from build123d import *

# Parameters (mm, degrees)
SKETCH1_W                = 36.8554
SKETCH1_H                = 17.1196
SKETCH1_W_2              = 19.8882
SKETCH1_H_2              = 6.985
SKETCH1_W_3              = 11.8237
SKETCH1_H_3              = 7.62
BOSS_EXTRUDE1_DEPTH      = 11.684
BOSS_EXTRUDE1_2_DEPTH    = 11.684
SKETCH3_R                = 1.4605
CUT_EXTRUDE8_DEPTH       = 140.210429827
SKETCH4_R                = 1.4605
CUT_EXTRUDE9_DEPTH       = 18.034
CUT_EXTRUDE11_DEPTH      = 38.1
SKETCH6_R                = 1.4605
CUT_EXTRUDE12_DEPTH      = 16.3195
CUT_EXTRUDE13_DEPTH      = 140.210429862
CUT_EXTRUDE13_DEPTH_BACK = 140.210429862
SKETCH7_R                = 1.9685
CUT_EXTRUDE14_DEPTH      = 7.62


with BuildPart() as part:
    # Sketch1 → Boss-Extrude1 (new body)
    with BuildSketch(Plane(origin=(0, 0, 0), x_dir=(1, 0, 0), z_dir=(0, 1, 0))):
        with BuildLine():
            Line((-25.4, 37.231859639), (-67.6656, 37.231859639))
            Line((-67.6656, 37.231859639), (-86.5378, 37.231859639))
            Line((-86.5378, 37.231859639), (-130.704860186, 33.167859639))
            Line((-130.704860186, 33.167859639), (-133.6294, 28.523199453))
            Line((-133.6294, 28.523199453), (-133.6294, 5.586999453))
            Line((-133.6294, 5.586999453), (-128.984739814, 2.662459639))
            Line((-128.984739814, 2.662459639), (-96.664183529, -1.34664073))
            ThreePointArc((-96.664183529, -1.34664073), (-60.341965715, -8.501620237), (-25.4, -20.730940361))
            Line((-25.4, -20.730940361), (-25.4, 37.231859639))
        make_face()
        with Locations((-111.1123, 17.953259639)):
            Rectangle(SKETCH1_W, SKETCH1_H, mode=Mode.SUBTRACT)
        with Locations((-76.367777447, 27.363959639)):
            Rectangle(SKETCH1_W_2, SKETCH1_H_2, mode=Mode.SUBTRACT)
        with Locations((-57.99455, 3.456462042)):
            Rectangle(SKETCH1_W_3, SKETCH1_H_3, mode=Mode.SUBTRACT)
        Polygon((-63.9064, 13.384739375), (-48.6664, 13.384739375), (-52.7304, 27.608739375), (-59.8424, 27.608739375), align=None, mode=Mode.SUBTRACT)
    extrude(amount=BOSS_EXTRUDE1_DEPTH)


with BuildPart() as body_2:
    # Sketch1 → Boss-Extrude1 2 (new body)
    with BuildSketch(Plane(origin=(0, 0, 0), x_dir=(1, 0, 0), z_dir=(0, 1, 0))):
        with BuildLine():
            Line((25.4, -20.730940361), (25.4, 37.231859639))
            Line((25.4, 37.231859639), (67.6656, 37.231859639))
            Line((67.6656, 37.231859639), (86.5378, 37.231859639))
            Line((86.5378, 37.231859639), (130.704860186, 33.167859639))
            Line((130.704860186, 33.167859639), (133.6294, 28.523199453))
            Line((133.6294, 28.523199453), (133.6294, 5.586999453))
            Line((133.6294, 5.586999453), (128.984739814, 2.662459639))
            Line((128.984739814, 2.662459639), (96.664183529, -1.34664073))
            ThreePointArc((96.664183529, -1.34664073), (60.341965715, -8.501620237), (25.4, -20.730940361))
        make_face()
        Polygon((59.8424, 27.608739375), (63.9064, 13.384739375), (48.6664, 13.384739375), (52.7304, 27.608739375), align=None, mode=Mode.SUBTRACT)
        with Locations((57.99455, 3.456462042)):
            Rectangle(SKETCH1_W_3, SKETCH1_H_3, mode=Mode.SUBTRACT)
        with Locations((76.367777447, 27.363959639)):
            Rectangle(SKETCH1_W_2, SKETCH1_H_2, mode=Mode.SUBTRACT)
        with Locations((111.1123, 17.953259639)):
            Rectangle(SKETCH1_W, SKETCH1_H, mode=Mode.SUBTRACT)
    extrude(amount=BOSS_EXTRUDE1_2_DEPTH)


with BuildPart() as cut_extrude8_tool:
    # Sketch3 → Cut-Extrude8 (new, through all)
    with BuildSketch(Plane.XY):
        with Locations((-127.524239814, 5.842)):
            Circle(SKETCH3_R)
        with Locations((127.524239814, 5.842)):
            Circle(SKETCH3_R)
    extrude(amount=-CUT_EXTRUDE8_DEPTH)


with BuildPart() as part_1:
    add(part.part)

    # Cut-Extrude8: cut by cut_extrude8_tool
    add(cut_extrude8_tool.part, mode=Mode.SUBTRACT)


with BuildPart() as body_2_1:
    add(body_2.part)

    # Cut-Extrude8: cut by cut_extrude8_tool
    add(cut_extrude8_tool.part, mode=Mode.SUBTRACT)


with BuildPart() as cut_extrude9_tool:
    # Sketch4 → Cut-Extrude9 (new body)
    with BuildSketch(Plane(origin=(0, 0, -37.231859639), x_dir=(-1, 0, 0), z_dir=(0, 0, -1))):
        with Locations((78.9178, 5.842)):
            Circle(SKETCH4_R)
        with Locations((-78.9178, 5.842)):
            Circle(SKETCH4_R)
    extrude(amount=-CUT_EXTRUDE9_DEPTH)


with BuildPart() as part_2:
    add(part_1.part)

    # Cut-Extrude9: cut by cut_extrude9_tool
    add(cut_extrude9_tool.part, mode=Mode.SUBTRACT)


with BuildPart() as body_2_2:
    add(body_2_1.part)

    # Cut-Extrude9: cut by cut_extrude9_tool
    add(cut_extrude9_tool.part, mode=Mode.SUBTRACT)

    # Sketch2 → Cut-Extrude11 (cut, symmetric)
    with BuildSketch(Plane.XY):
        with BuildLine():
            Line((25.4, 5.842), (25.4, 0))
            Line((25.4, 0), (31.242, 0))
            ThreePointArc((31.242, 0), (27.111082184, 1.711082184), (25.4, 5.842))
        make_face()
        with BuildLine():
            Line((25.4, 11.684), (25.4, 5.842))
            ThreePointArc((25.4, 5.842), (27.111082184, 9.972917816), (31.242, 11.684))
            Line((31.242, 11.684), (25.4, 11.684))
        make_face()
    extrude(amount=CUT_EXTRUDE11_DEPTH, both=True, mode=Mode.SUBTRACT)

    # Sketch6 → Cut-Extrude12 (cut, symmetric)
    with BuildSketch(Plane.XY):
        with Locations((57.6326, 5.842)):
            Circle(SKETCH6_R)
    extrude(amount=CUT_EXTRUDE12_DEPTH, both=True, mode=Mode.SUBTRACT)

    # Sketch7 → Cut-Extrude13 (cut, two sides: drawn at the far end of the back side and taken through both)
    with BuildSketch(Plane.XY.offset(-CUT_EXTRUDE13_DEPTH_BACK)):
        with Locations((31.242, 5.842)):
            Circle(SKETCH7_R)
    extrude(amount=CUT_EXTRUDE13_DEPTH + CUT_EXTRUDE13_DEPTH_BACK, mode=Mode.SUBTRACT)

    # Sketch8 → Cut-Extrude14 (cut)
    with BuildSketch(Plane.XZ):
        with BuildLine():
            Line((34.870867511, 3.534001348), (24.218880791, 9.085239089))
            Line((24.218880791, 9.085239089), (24.658356534, -12.669081964))
            Line((24.658356534, -12.669081964), (33.631457802, -9.925148709))
            ThreePointArc((33.631457802, -9.925148709), (38.767733035, -3.611490076), (34.870867511, 3.534001348))
        make_face()
    extrude(amount=-CUT_EXTRUDE14_DEPTH, mode=Mode.SUBTRACT)


solid = body_2_2.part
Could you check a few things on this model? Use its own coordinates, in mm. A direction names the side the tool comes from. Give positions to 0.01 mm unless a question says otherwise; leave off trailing zeros. Loops run counter-clockwise (first coordinate to the right, second up) from the corner with the lowest first, then second, coordinate; pieces in that order, holes last. Notation, with made-up numbers: M -5,8 L 28,8 A26 cw 28,39 Z; hole C -14.75,66.5 d7. An arc over 180 degrees is marked long. Answer as a JSON object with one key per item and string values.
Q1. For faces 1 (the flat face through (56, 6, -37.232)), 2 (the cylindrical face through (77.57, 5.28, -34.09)), 3 (the flat face through (59, 7, -7.266)), 4 (the cylindrical face through (126.065, 5.906, -5.789)), 5 (the flat face through (30.2, 3.76, 5.97)), which set-ups out of +Z, -Z, +X, -X, +Y, -Y let a thin tool reach every point of the face, with its end or its side?
Values found:
{"face 1": "-Z, +X, -X, +Y, -Y", "face 2": "-Z", "face 3": "+Y, -Y", "face 4": "+Z, -Z", "face 5": "-X, -Y"}
Q2. Suppose I cut it at C-C, the plane x = 95. List the corners of the cut face in (y, z) for me, plus the area to 3 significant figures.
Values found:
{"outline": "M 0,-36.45 L 11.68,-36.45 L 11.68,-26.51 L 0,-26.51 Z; M 0,-9.39 L 11.68,-9.39 L 11.68,1.56 L 0,1.56 Z", "area": "244 mm²"}
Q3. If I drill on probe 1 along Z at (x, y) = (82.5, 7); probe 2 along Z at (x, y) = (59, 7.25); probe 3 along X at (y, z) = (9.25, -14), over which ranges is the centre line in solid material (lowest first)? Write a range as [from, to].
Values found:
{"probe 1": "z = [-37.23, -30.86], [-23.87, 3.5]", "probe 2": "z = [-37.23, -27.61], [-13.38, -7.27], [0.35, 8.87]", "probe 3": "x = [26.5, 48.84], [63.73, 92.68], [129.54, 133.63]"}
Q4. For P1, Ø2, axis at x = 74.5, y = 5.5, coming from the +Z side; P2, Ø4.5, axis at x = 127.52, y = 5.84, coming from the -Z side; P3, Ø1.5, axis at x = 69, y = 3, coming from the +Z side, each with a flat end and sliding along its axis, tell me the tip position at first contact or that it passes through.
Values found:
{"P1": "stops at z = 5.29", "P2": "stops at z = -33.67", "P3": "stops at z = 6.48"}
Q5. Suppose I cut it at A-A, the plane x = 114.5. List the corners of the cut face in (y, z) for me.
Values found:
{"outline": "M 0,-34.66 L 11.68,-34.66 L 11.68,-26.51 L 0,-26.51 Z; M 0,-9.39 L 11.68,-9.39 L 11.68,-0.87 L 0,-0.87 Z"}
Q6. Suppose I cut it at D-D, the plane x = 45.5. List the corners of the cut face in (y, z) for me.
Values found:
{"outline": "M 0,-37.23 L 11.68,-37.23 L 11.68,13.02 L 0,13.02 Z"}
Q7. Suppose I cut it at B-B, the plane y = 2.75. List the corners of the cut face in (x, z) for me (1 decimal).
Values found:
{"outline": "M 26.3,-37.2 L 86.5,-37.2 L 130.7,-33.2 L 133.6,-28.5 L 133.6,-5.6 L 129,-2.7 L 96.7,1.3 A260.6 cw 26.3,20.4 L 26.3,8 L 34.9,3.5 A7.3 cw 33.6,-9.9 L 26.3,-12.2 Z; hole M 48.7,-13.4 L 52.7,-27.6 L 59.8,-27.6 L 63.9,-13.4 Z; hole M 52.1,-7.3 L 63.9,-7.3 L 63.9,0.4 L 52.1,0.4 Z; hole M 66.4,-30.9 L 86.3,-30.9 L 86.3,-23.9 L 66.4,-23.9 Z; hole M 92.7,-26.5 L 129.5,-26.5 L 129.5,-9.4 L 92.7,-9.4 Z"}
Q8. If we mould it in two halves opening along X, with no side actions, what happens to faces 6 (the flat face through (108.31, 5.76, -35.23)), 7 (the flat face through (29.46, 3.76, -11.2)), 8 (the flat face through (92.685, 6, -18))? For each: pulls with the +X half, pulls with the -X half, needs draft (parallel to the pull), parting line crosses it, or undercut.
Values found:
{"face 6": "pulls with the +X half", "face 7": "pulls with the -X half", "face 8": "undercut"}
